Verification items for this drawing (mm, ordinates from the low corner). Give positions to 0.01 mm unless a question says otherwise; leave off trailing zeros. Loops run counter-clockwise (first coordinate to the right, second up) from the corner with the lowest first, then second, coordinate; pieces in that order, holes last. Notation, with made-up numbers: M 76,30 L 96,30 A20 ccw 96,34 Z; hole C 38,26.5 d3. An arc over 180 degrees is marked long. Answer in a Markdown table with one row per item.
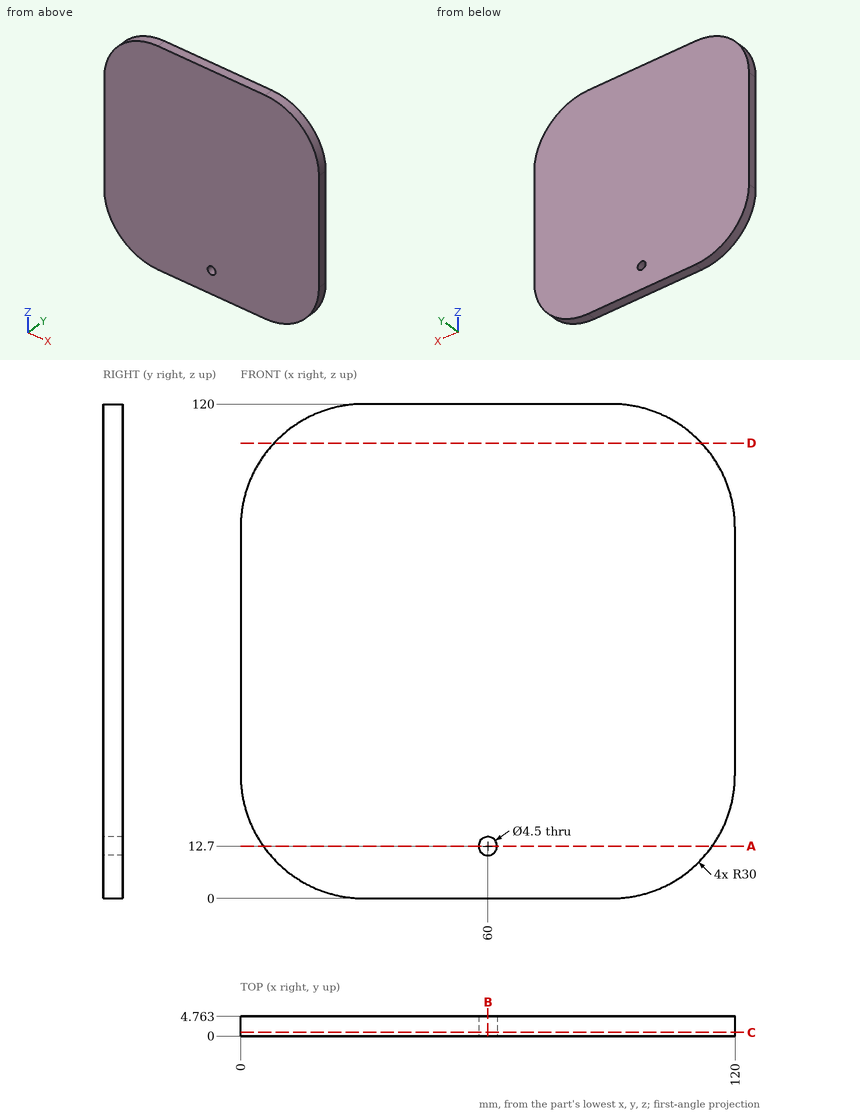
Item 1: Sectioned sample at B-B (x = 60). Record the cut outline in (y, z), and give its area (3 significant figures).
Reported:
| item | result |
|---|---|
| outline | M 0,0 L 4.76,0 L 4.76,10.45 L 0,10.45 Z; M 0,14.95 L 4.76,14.95 L 4.76,120 L 0,120 Z |
| area | 550 mm^2 |
Item 2: Sectioned sample at C-C (y = 0.9). Record the cut outline in (x, z).
Reported:
| item | result |
|---|---|
| outline | M 0,30 A30 ccw 30,0 L 90,0 A30 ccw 120,30 L 120,90 A30 ccw 90,120 L 30,120 A30 ccw 0,90 Z; hole C 60,12.7 d4.5 |
Item 3: Sectioned sample at A-A (z = 12.7). Record the cut outline in (x, y).
Reported:
| item | result |
|---|---|
| outline | M 5.49,0 L 57.75,0 L 57.75,4.76 L 5.49,4.76 Z; M 62.25,0 L 114.51,0 L 114.51,4.76 L 62.25,4.76 Z |
Item 4: Go/stop test with a flat-tipped pin: pin 1 (1.5 mm diameter, centred on y = 1.5, z = 102.5, fed in from -X). Record where the tip stops, or that it passes through.
Reported:
| item | result |
|---|---|
| pin 1 | stops at x = 2.4 |
Item 5: Sectioned sample at D-D (z = 110.5). Record the cut outline in (x, y).
Reported:
| item | result |
|---|---|
| outline | M 8.1,0 L 111.9,0 L 111.9,4.76 L 8.1,4.76 Z |
Item 6: Scan lines: L1, parallel to Z at x = 60, y = 1.8; L2, parallel to X at y = 4.5, z = 28.5; L3, parallel to Z at x = 27, y = 0.85. Record each from-to range of solid material in increasing order. Write a range as [from, to].
Reported:
| item | result |
|---|---|
| L1 | z = [0, 10.45], [14.95, 120] |
| L2 | x = [0.04, 119.96] |
| L3 | z = [0.15, 119.85] |
